Verification items for the finished model (mm, model axes). A direction names the side the tool comes from. Coordinates: 2 decimals unless noted, no trailing zeros. Order: outer loops, then holes, each group sorted by start corner. A loop starts at its lowest first (then second) coordinate and runs counter-clockwise, first axis right, second up.
Q1. Draft check along X on faces 3 (the flat face through (0, -17.5, 1)), 4 (the flat face through (-27.5, 0, 1)), 5 (the flat face through (-22.5, -11, 2)). Enter one of: pulls with the +X half, pulls with the -X half, needs draft (parallel to the pull), parting line crosses it, or undercut.
Q2. Depth check by flat-ended pin: P1, Ø1.3, axis at x = 10.52, y = -0.01, coming from the -Z side; P2, Ø10, axis at x = -18.5, y = 0, coming from the +Z side. Enter the tip coordinate at first touch or a pass-through.
Q3. Thickness scan on line 1 (Y direction, x = 0, z = 0.9); line 2 (Y direction, x = -18.6, z = 0.95); line 3 (Y direction, x = 16, z = 2). Record the ranges inside material, lowest first.
Q4. Set-up check for faces 1 (the flat face through (-19.5, -11, 2)), 2 (the flat face through (0, 4, 3)): record each of +Z, -Z, +X, -X, +Y, -Y from which the full face is reachable in a straight line by a thin tool's end or side.
Q5. Cross-section at A-A, the plane x = -18.6. Record the boundary of the cut face in (y, z), and give its area (3 significant figures).
Q6. Cross-section at B-B, the plane z = 0.85. Count the separate pieces of the cut face and the enclosed holes in it, and give its area (3 significant figures).
from build123d import *

# Parameters (mm, degrees)
SKETCH1_W           = 55
SKETCH1_H           = 35
SKETCH1_R           = 1.5
SKETCH1_R_2         = 0.5
BOSS_EXTRUDE1_DEPTH = 3
SKETCH2_W           = 25
SKETCH2_H           = 2
CUT_EXTRUDE1_DEPTH  = 4
SKETCH3_W           = 3
SKETCH3_H           = 3
CUT_EXTRUDE2_DEPTH  = 3
SKETCH4_R           = 1.047817358
SKETCH4_R_2         = 1.044805948
CUT_EXTRUDE3_DEPTH  = 3
SKETCH5_R           = 1.037971053
SKETCH5_R_2         = 1.052489193
CUT_EXTRUDE4_DEPTH  = 3


with BuildPart() as part:
    # Sketch1 → Boss-Extrude1 (new body)
    with BuildSketch(Plane.XY):
        Rectangle(SKETCH1_W, SKETCH1_H)
        with Locations((18.6, 0)):
            Circle(SKETCH1_R, mode=Mode.SUBTRACT)
        with Locations(Location((-18.6, 0, 0), (0, 0, 180))):
            Circle(SKETCH1_R, mode=Mode.SUBTRACT)
        Circle(SKETCH1_R_2, mode=Mode.SUBTRACT)
    extrude(amount=BOSS_EXTRUDE1_DEPTH)

    # Sketch2 → Cut-Extrude1 (cut)
    with BuildSketch(Plane.XY.offset(3)):
        with Locations((0.008423928, -12)):
            Rectangle(SKETCH2_W, SKETCH2_H)
    extrude(amount=-CUT_EXTRUDE1_DEPTH, mode=Mode.SUBTRACT)

    # Sketch3 → Cut-Extrude2 (cut)
    with BuildSketch(Plane.XY.offset(3)):
        with Locations((-21, -11)):
            Rectangle(SKETCH3_W, SKETCH3_H)
        with Locations((-15, -11)):
            Rectangle(SKETCH3_W, SKETCH3_H)
        with Locations((15, -11)):
            Rectangle(SKETCH3_W, SKETCH3_H)
        with Locations((21, -11)):
            Rectangle(SKETCH3_W, SKETCH3_H)
    extrude(amount=-CUT_EXTRUDE2_DEPTH, mode=Mode.SUBTRACT)

    # Sketch4 → Cut-Extrude3 (cut)
    with BuildSketch(Plane.XY.offset(3)):
        with Locations((-10.502321648, -0.002631042)):
            Circle(SKETCH4_R)
        with Locations((10.523984619, -0.009290749)):
            Circle(SKETCH4_R_2)
    extrude(amount=-CUT_EXTRUDE3_DEPTH, mode=Mode.SUBTRACT)

    # Sketch5 → Cut-Extrude4 (cut)
    with BuildSketch(Plane.XY.offset(3)):
        with Locations((-10.504210452, 12.485998178)):
            Circle(SKETCH5_R)
        with Locations((10.494217, 12.488375227)):
            Circle(SKETCH5_R_2)
    extrude(amount=-CUT_EXTRUDE4_DEPTH, mode=Mode.SUBTRACT)


solid = part.part
Check values:
1. face 3: needs draft
1. face 4: pulls with the -X half
1. face 5: undercut
2. P1: passes through
2. P2: stops at z = 3
3. line 1: y = -17.5 to -13, -11 to -0.5, 0.5 to 17.5
3. line 2: y = -17.5 to -1.5, 1.5 to 17.5
3. line 3: y = -17.5 to -12.5, -9.5 to 17.5
4. face 1: +Z, -Z
4. face 2: +Z, +X, -X, +Y, -Y
5. outline: (-17.5, 0) - (-1.5, 0) - (-1.5, 3) - (-17.5, 3) - close; (1.5, 0) - (17.5, 0) - (17.5, 3) - (1.5, 3) - close
5. area: 96.0 mm2
6. separate pieces: 1
6. enclosed holes: 12
6. area: 1,810 mm2
